from build123d import *

# Parameters (mm, degrees)
CLAMP_EXTRUDE_DEPTH     = 10
HOLE_R                  = 1.5
HOLES_CUT_EXTRUDE_DEPTH = 4
FILLET1_R               = 1


with BuildPart() as part:
    # Sketch4 → Clamp Extrude (new body)
    with BuildSketch(Plane(origin=(0, 0, 0), x_dir=(0, 0, -1), z_dir=(1, 0, 0))):
        with BuildLine():
            Line((-23.6125, 0), (-11.1125, 0))
            ThreePointArc((-11.1125, 0), (0, -11.1125), (11.1125, 0))
            Line((11.1125, 0), (23.6125, 0))
            Line((23.6125, 0), (23.6125, -3))
            Line((23.6125, -3), (13.789947652, -3))
            ThreePointArc((13.789947652, -3), (0, -14.1125), (-13.789947652, -3))
            Line((-13.789947652, -3), (-23.6125, -3))
            Line((-23.6125, -3), (-23.6125, 0))
        make_face()
    extrude(amount=CLAMP_EXTRUDE_DEPTH)

    # Hole → Holes Cut-Extrude (cut, through all)
    with BuildSketch(Plane.XZ.offset(3)):
        with Locations((5, 18.701223826)):
            Circle(HOLE_R)
        with Locations((5, -18.701223826)):
            Circle(HOLE_R)
    extrude(amount=-HOLES_CUT_EXTRUDE_DEPTH, mode=Mode.SUBTRACT)

    # Fillet1
    fillet1_edges = [part.edges().sort_by_distance(p)[0] for p in [
        (0, -1.5, -23.6125),
        (0, -3, -18.701223826),
        (0, -14.1125, 0),
        (10, -1.5, -23.6125),
        (5, -3, 13.789947652),
        (5, -3, 23.6125),
        (5, -3, -23.6125),
        (5, -3, -13.789947652),
        (10, -1.5, 23.6125),
        (10, -3, 18.701223826),
        (10, -14.1125, 0),
        (0, -3, 18.701223826),
        (10, -3, -18.701223826),
        (0, -1.5, 23.6125),
    ]]
    fillet(fillet1_edges, radius=FILLET1_R)


solid = part.part
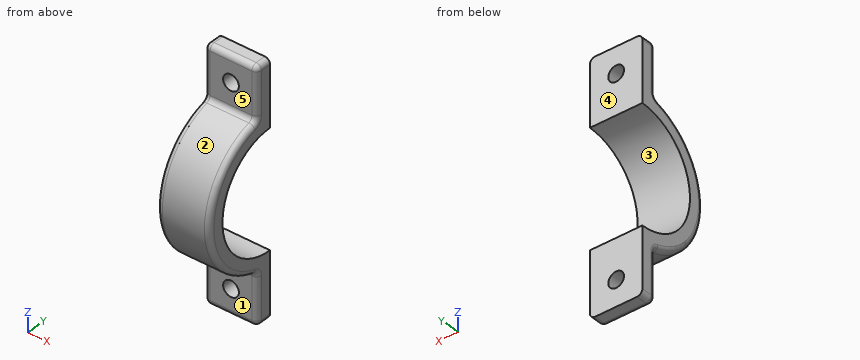
Source: CAD feature listing. Evaluate the final solid. Frame: model axes, mm. Face numbers are marked on the shaded views. A direction names the side the tool comes from. Coordinates: 2 decimals unless noted, no trailing zeros. Write each loop counter-clockwise with the first axis right and the second up, starting at its lowest first coordinate (ties: lowest second). Pieces come first, ordered by that corner, then holes. Notation, with made-up numbers: M 43,3.5 L 53,3.5 A11 cw 53,20.5 Z; hole C 43.25,15 d8. An arc over 180 degrees is marked long. Use a Markdown table: item, result.
1) First-contact query: pin 1 Ø2 at (x, y) = (3, -6.5) entering from -Z; pin 2 Ø6 at (x, z) = (2.5, 4) entering from -Y; pin 3 Ø4 at (x, y) = (5, -12.5) entering from +Z; pin 4 Ø8 at (y, z) = (-4, -8) entering from -X. Flat tips, straight axial feed; report the tip coordinate or a pass-through.
Conclusion:
| item | result |
|---|---|
| pin 1 | stops at z = -13 |
| pin 2 | stops at y = -14.08 |
| pin 3 | stops at z = 9.43 |
| pin 4 | stops at x = 0 |
2) Section C-C, the plane z = 0. Output: boundary loops of the cut face in (x, y).
Conclusion:
| item | result |
|---|---|
| outline | M 0,-13.11 A1 ccw 1,-14.11 L 9,-14.11 A1 ccw 10,-13.11 L 10,-11.11 L 0,-11.11 Z |
3) Section A-A, the plane x = 5. Output: boundary loops of the cut face in (y, z) (1 decimal), then the cut area to 3 significant figures.
Conclusion:
| item | result |
|---|---|
| outline | M -3.7,-13.6 A1 cw -3,-14.6 L -3,-17.2 L 0,-17.2 L 0,-11.1 A11.1 cw 0,11.1 L 0,17.2 L -3,17.2 L -3,14.6 A1 cw -3.7,13.6 A14.1 ccw Z; M -3,-22.6 A1 ccw -2,-23.6 L 0,-23.6 L 0,-20.2 L -3,-20.2 Z; M -3,20.2 L 0,20.2 L 0,23.6 L -2,23.6 A1 ccw -3,22.6 Z |
| area | 158 mm^2 |
4) Mould query, pull axis Z, two halves, no side actions, for the marked faces 1, 2 and 3. Classes: pulls with the +Z half, pulls with the -Z half, needs draft (parallel to the pull), parting line crosses it, or undercut.
Conclusion:
| item | result |
|---|---|
| face 1 | needs draft |
| face 2 | parting line crosses it |
| face 3 | undercut |
5) Section D-D, the plane x = 0.5. Output: boundary loops of the cut face in (y, z) (1 decimal).
Conclusion:
| item | result |
|---|---|
| outline | M -3.7,-13.5 A1.1 cw -2.9,-14.6 L -2.9,-22.6 A0.9 ccw -2,-23.5 L 0,-23.5 L 0,-11.1 A11.1 cw 0,11.1 L 0,23.5 L -2,23.5 A0.9 ccw -2.9,22.6 L -2.9,14.6 A1.1 cw -3.7,13.5 A14 ccw Z |
6) Reachability of the marked faces 4 and 5 from +Z, -Z, +X, -X, +Y, -Y: full face, straight path, thin tool, end or side. Return the list, or none.
Conclusion:
| item | result |
|---|---|
| face 4 | +Z, -Z, +X, -X, +Y |
| face 5 | +Z, +X, -X, -Y |
7) Section B-B, the plane x = 7.5. Output: boundary loops of the cut face in (y, z) (1 decimal), then the cut area to 3 significant figures.
Conclusion:
| item | result |
|---|---|
| outline | M -3.7,-13.6 A1 cw -3,-14.6 L -3,-22.6 A1 ccw -2,-23.6 L 0,-23.6 L 0,-11.1 A11.1 cw 0,11.1 L 0,23.6 L -2,23.6 A1 ccw -3,22.6 L -3,14.6 A1 cw -3.7,13.6 A14.1 ccw Z |
| area | 176 mm^2 |
8) Ray query, L1, parallel to Z at x = 5, y = -1.85; L2, parallel to Z at x = 5, y = -1.95; L3, parallel to Y at x = 2.25, z = 17. Return the intervals inside material, ascending.
Conclusion:
| item | result |
|---|---|
| L1 | z = -23.61 to -20.2, -17.2 to -10.96, 10.96 to 17.2, 20.2 to 23.61 |
| L2 | z = -23.61 to -20.2, -17.2 to -10.94, 10.94 to 17.2, 20.2 to 23.61 |
| L3 | y = -3 to 0 |
